Read the model definition and answer for the solid it produces. Units are mm, in the model's axes. A direction names the side the tool comes from. Coordinates: 2 decimals unless noted, no trailing zeros. Order: outer loops, then holes, each group sorted by start corner. A loop starts at its lowest first (then second) coordinate and runs counter-clockwise, first axis right, second up. Notation, with made-up numbers: (-15.75, -23.75) - (-10.75, -23.75) arc R26 ccw to (-10.75, 7.25) - close; hole circle Ø11 at (-18, 54). An arc over 180 degrees is marked (long way). Write item = value, one per line.
from build123d import *

# Parameters (mm, degrees)
F1_DEPTH = 63.5
F0_W     = 25.4
F0_H     = 19.05
F2_DEPTH = 25.4
F3_DEPTH = 7.9375
F5_R     = 5.08
F6_DEPTH = 25.4
F7_DEPTH = 25.4
F8_DEPTH = 304.8


with BuildPart() as f1:
    # F0 (on Front) → F1 (new body, symmetric)
    with BuildSketch(Plane.XZ):
        Polygon((22.225, 9.525), (-41.275, 9.525), (-41.275, -9.525), (41.275, -9.525), (41.275, 9.525), align=None)
    extrude(amount=F1_DEPTH, both=True)

    # F0 (on Front) → F2 (join, symmetric)
    with BuildSketch(Plane.XZ):
        with BuildLine():
            Line((22.225, 27.0002), (22.225, 9.525))
            Line((22.225, 9.525), (41.275, 9.525))
            Line((41.275, 9.525), (41.275, 27.0002))
            ThreePointArc((41.275, 27.0002), (45.9246798487, 38.2255201513), (57.15, 42.8752))
            Line((57.15, 42.8752), (60.325, 42.8752))
            Line((60.325, 42.8752), (60.325, 61.9252))
            Line((60.325, 61.9252), (57.15, 61.9252))
            add(Edge.make_bspline(
                [(53.8854342407, 61.7722898912), (54.9842067368, 61.8365871986), (56.0728453275, 61.8876096574), (57.15, 61.9252)],
                knots=[108.5245810491, 108.5245810491, 108.5245810491, 108.5245810491, 111.5045361635, 111.5045361635, 111.5045361635, 111.5045361635], degree=3))
            ThreePointArc((53.8854342407, 61.7722898912), (31.3258777096, 50.5133948686), (22.225, 27.0002))
        make_face()
        with Locations((73.025, 52.4002)):
            Rectangle(F0_W, F0_H)
    extrude(amount=F2_DEPTH, both=True)

    # F0 (on Front) → F3 (join, symmetric)
    with BuildSketch(Plane.XZ):
        with BuildLine():
            add(Edge.make_bspline(
                [(-41.275, 9.525), (-39.5856284224, 39.4828766469), (13.870125209, 59.4306981306), (53.8854342407, 61.7722898912)],
                knots=[0, 0, 0, 0, 108.5245810491, 108.5245810491, 108.5245810491, 108.5245810491], degree=3))
            Line((-41.275, 9.525), (22.225, 9.525))
            Line((22.225, 9.525), (22.225, 27.0002))
            ThreePointArc((22.225, 27.0002), (31.3258777096, 50.5133948686), (53.8854342407, 61.7722898912))
        make_face()
    extrude(amount=F3_DEPTH, both=True)

    # F0 (on Front) → F4 (revolve)
    with BuildSketch(Plane.XZ):
        Polygon((85.725, 66.675), (85.725, 61.9252), (85.725, 42.8752), (85.725, 38.1), (111.125, 38.1), (111.125, 66.675), align=None)
    revolve(axis=Axis((85.725, 0, 52.3875), (0, 0, 1)))

    # F5
    f5_edges = [f1.edges().sort_by_distance(p)[0] for p in [
        (41.275, -63.5, 0),
        (-41.275, -63.5, 0),
        (41.275, 63.5, 0),
        (-41.275, 63.5, 0),
    ]]
    fillet(f5_edges, radius=F5_R)

    # F6 (add): a face of the model
    f6_faces = [f1.faces().sort_by_distance(p)[0] for p in [
        (85.725, 0, 66.675),
    ]]
    extrude(f6_faces, amount=F6_DEPTH)

    # F7 (add): faces of the model
    f7_faces = [f1.faces().sort_by_distance(p)[0] for p in [
        (48.8772671015, -25.4, 41.5257592525),
        (0, -63.5, 0),
    ]]
    extrude(f7_faces, amount=F7_DEPTH)

    # F8 (add): a face of the model
    f8_faces = [f1.faces().sort_by_distance(p)[0] for p in [
        (0, -11.3906341446, -9.525),
    ]]
    extrude(f8_faces, amount=F8_DEPTH)


solid = f1.part
1) Flat-ended cylindrical pins translate along their axes: pin 1 Ø14 at (y, z) = (14, 19) entering from -X; pin 2 Ø5.5 at (y, z) = (-73.5, -3.5) entering from +X (3 decimals); pin 3 Ø5 at (y, z) = (-28, 21) entering from -X (3 decimals); pin 4 Ø12 at (x, z) = (49.5, -108.5) entering from +Y. Find the tip coordinate at first contact, or state that the pin passes through.
Returned:
pin_1 = -40.23
pin_2 = 36.195
pin_3 = 22.225
pin_4 = through
2) Straight lines are drawn through the part: line 1 along Z through (x, y) = (-17, -33.5) (3 decimals); line 2 along X through (y, z) = (-53, -149) (3 decimals); line 3 along Y through (x, z) = (17, 16). For each, find the intervals that lie inside material, in ascending order. Write a range as from..to.
Returned:
line_1 = -314.325..9.525
line_2 = -41.275..41.275
line_3 = -7.94..7.94
3) The part is cut by section D-D (y = 53). Determine the outline of the cut face in (x, z) (3 decimals), and give its area (3 significant figures).
Returned:
outline = (-41.275, -314.325) - (41.275, -314.325) - (41.275, 9.525) - (-41.275, 9.525) - close
area = 26,700 mm^2
4) Determine the mould class of faces 4 (the face through (46, -50.8, 42)), 5 (the face through (68, -21, 42.875)), 6 (the face through (-41.275, 1, -150)) for opening direction X: pulls with the +X half, pulls with the -X half, needs draft (parallel to the pull), parting line crosses it, or undercut.
Returned:
face_4 = needs draft
face_5 = undercut
face_6 = pulls with the -X half
5) The part is cut by section A-A (z = -106.5). Determine the outline of the cut face in (x, y) (3 decimals).
Returned:
outline = (-41.275, -58.42) arc R5.08 ccw to (-36.195, -63.5) - (-36.195, -88.9) - (36.195, -88.9) - (36.195, -63.5) arc R5.08 ccw to (41.275, -58.42) - (41.275, 58.42) arc R5.08 ccw to (36.195, 63.5) - (-36.195, 63.5) arc R5.08 ccw to (-41.275, 58.42) - close
6) The part is cut by section B-B (x = 65). Determine the outline of the cut face in (y, z) (1 decimal).
Returned:
outline = (-50.8, 42.9) - (-14.7, 42.9) - (-14.7, 38.1) - (14.7, 38.1) - (14.7, 42.9) - (25.4, 42.9) - (25.4, 61.9) - (14.7, 61.9) - (14.7, 92.1) - (-14.7, 92.1) - (-14.7, 61.9) - (-50.8, 61.9) - close
7) For faces 1 (the face through (85.725, -38, 52)), 2 (the face through (31.57, -29.07, 50.78)), 3 (the face through (86, 0, 38.1)), determine the directions among +Z, -Z, +X, -X, +Y, -Y from which every point of the face is accessible in a straight line to the end or side of a thin tool.
Returned:
face_1 = +Z, -Z, +X, -Y
face_2 = +Z, -X, -Y
face_3 = -Z, +X, +Y, -Y
8) The part is cut by section C-C (y = -78). Determine the outline of the cut face in (x, z) (3 decimals).
Returned:
outline = (-36.195, -314.325) - (36.195, -314.325) - (36.195, 9.525) - (-36.195, 9.525) - close
